from build123d import *

# Parameters (mm, degrees)
SKETCH1_W           = 49.022
SKETCH1_H           = 101.6
BOSS_EXTRUDE1_DEPTH = 7.62
SKETCH2_R           = 5.08
CUT_EXTRUDE1_DEPTH  = 7.62
SKETCH4_W           = 49.022
SKETCH4_H           = 29.845
CUT_EXTRUDE2_DEPTH  = 57.916548745
SKETCH5_R           = 1.905
CUT_EXTRUDE3_DEPTH  = 17.78
BOSS_EXTRUDE3_START = 25.4
SKETCH6_R           = 1.905
BOSS_EXTRUDE3_DEPTH = 25.4


with BuildPart() as part:
    # Sketch1 → Boss-Extrude1 (new body)
    with BuildSketch(Plane(origin=(0, 0, 0), x_dir=(1, 0, 0), z_dir=(0, 1, 0))):
        Rectangle(SKETCH1_W, SKETCH1_H)
    extrude(amount=BOSS_EXTRUDE1_DEPTH)

    # Sketch2 → Cut-Extrude1 (cut)
    with BuildSketch(Plane(origin=(0, 7.62, 0), x_dir=(1, 0, 0), z_dir=(0, 1, 0))):
        with Locations(Location((12.7, -34.29, 0), (0, 0, 270))):
            Circle(SKETCH2_R)
        with Locations(Location((-12.7, -34.29, 0), (0, 0, 270))):
            Circle(SKETCH2_R)
    extrude(amount=-CUT_EXTRUDE1_DEPTH, mode=Mode.SUBTRACT)

    # Sketch4 → Cut-Extrude2 (cut, through all)
    with BuildSketch(Plane(origin=(0, 7.62, 0), x_dir=(1, 0, 0), z_dir=(0, 1, 0))):
        with Locations((0, 35.8775)):
            Rectangle(SKETCH4_W, SKETCH4_H)
    extrude(amount=-CUT_EXTRUDE2_DEPTH, mode=Mode.SUBTRACT)

    # Sketch5 → Cut-Extrude3 (cut)
    with BuildSketch(Plane(origin=(0, 0, -20.955), x_dir=(-1, 0, 0), z_dir=(0, 0, -1))):
        with Locations((-16.891, 3.81)):
            Circle(SKETCH5_R)
        with Locations((-7.62, 3.81)):
            Circle(SKETCH5_R)
        with Locations((7.62, 3.81)):
            Circle(SKETCH5_R)
        with Locations((16.891, 3.81)):
            Circle(SKETCH5_R)
    extrude(amount=-CUT_EXTRUDE3_DEPTH, mode=Mode.SUBTRACT)

    # Sketch6 → Boss-Extrude3 (add)
    with BuildSketch(Plane(origin=(0, 0, -3.175), x_dir=(-1, 0, 0), z_dir=(0, 0, -1)).offset(BOSS_EXTRUDE3_START)):
        with Locations((-16.891, 3.81)):
            Circle(SKETCH6_R)
        with Locations((16.891, 3.81)):
            Circle(SKETCH6_R)
    extrude(amount=-BOSS_EXTRUDE3_DEPTH)


solid = part.part
Verification items for the finished model (mm, model axes). A direction names the side the tool comes from. Give positions to 0.01 mm unless a question says otherwise; leave off trailing zeros. Loops run counter-clockwise (first coordinate to the right, second up) from the corner with the lowest first, then second, coordinate; pieces in that order, holes last.
1. Cross-section at D-D on y = 3.81. Record the cut outline in (x, z) (3 decimals).
Derived:
outline: (-24.511, -20.955) - (-18.796, -20.955) - (-18.796, -28.575) - (-14.986, -28.575) - (-14.986, -20.955) - (-9.525, -20.955) - (-9.525, -3.175) - (-5.715, -3.175) - (-5.715, -20.955) - (5.715, -20.955) - (5.715, -3.175) - (9.525, -3.175) - (9.525, -20.955) - (14.986, -20.955) - (14.986, -28.575) - (18.796, -28.575) - (18.796, -20.955) - (24.511, -20.955) - (24.511, 50.8) - (-24.511, 50.8) - close; hole circle Ø10.16 at (-12.7, 34.29); hole circle Ø10.16 at (12.7, 34.29)
2. Material ranges on probe 1 along X at (y, z) = (5, 34.29); probe 2 along X at (y, z) = (2.5, 38); probe 3 along Y at (x, z) = (-7.62, -7.25) (3 decimals), recorded low to high.
Derived:
probe 1: x = -24.51 to -17.78, -7.62 to 7.62, 17.78 to 24.51
probe 2: x = -24.51 to -16.17, -9.23 to 9.23, 16.17 to 24.51
probe 3: y = 0 to 1.905, 5.715 to 7.62
3. Cross-section at B-B on x = -12.7. Record the cut outline in (y, z) (3 decimals).
Derived:
outline: (0, -20.955) - (7.62, -20.955) - (7.62, 29.21) - (0, 29.21) - close; (0, 39.37) - (7.62, 39.37) - (7.62, 50.8) - (0, 50.8) - close
4. Go/stop test with flat-tipped pins: P1, Ø1.9, axis at x = -8, y = 3, coming from the -Z side (3 decimals); P2, Ø2.5, axis at x = 4.5, y = 2.5, coming from the -Z side (3 decimals); P3, Ø6, axis at x = -12.7, z = 34.29, coming from the -Y side; P4, Ø10, axis at x = -9.5, z = 1.5, coming from the -Y side. Record where each tip stops, or that it passes through.
Derived:
P1: stops at z = -3.175
P2: stops at z = -20.955
P3: passes through
P4: stops at y = 0
5. Tool access check on faces 1 (the flat face through (0, 4, 50.8)), 2 (the cylindrical face through (-18.71, 4.38, -24.82)). Record the directions out of +Z, -Z, +X, -X, +Y, -Y that give a thin tool (end or side, any length) a straight path to the whole face; none if there is none.
Derived:
face 1: +Z, +X, -X, +Y, -Y
face 2: -Z
6. Release check for a two-part mould opening along Y. For faces 3 (the flat face through (0, 0, 14)), 4 (the flat face through (-17, 4, -28.575)), 5 (the flat face through (-8, 4, -3.175)), 6 (the cylindrical face through (-9.437, 4.382, -12.189)) record: +Y half, -Y half, draft (parallel to the pull), parting line (faces both ways), or undercut.
Derived:
face 3: -Y half
face 4: draft
face 5: undercut
face 6: undercut
7. Cross-section at A-A on z = 34.29. Record the cut outline in (x, y).
Derived:
outline: (-24.51, 0) - (-17.78, 0) - (-17.78, 7.62) - (-24.51, 7.62) - close; (-7.62, 0) - (7.62, 0) - (7.62, 7.62) - (-7.62, 7.62) - close; (17.78, 0) - (24.51, 0) - (24.51, 7.62) - (17.78, 7.62) - close
8. Cross-section at C-C on z = -19. Record the cut outline in (x, y) (3 decimals).
Derived:
outline: (-24.511, 0) - (24.511, 0) - (24.511, 7.62) - (-24.511, 7.62) - close; hole circle Ø3.81 at (-7.62, 3.81); hole circle Ø3.81 at (7.62, 3.81)
